Can you work these out from the model? Positions are in its coordinate system, mm. A direction names the side the tool comes from. Coordinates: 2 decimals unless noted, no trailing zeros. Write each loop counter-clockwise with the first axis right and the second up, starting at its lowest first coordinate (ties: lowest second). Pieces come first, ordered by that corner, then holes.
Solid Edge part; units mm, degrees
sketch "Sketch1" plane through (0, 0, 0) normal (1, 0, 0) x (0, 1, 0)
  line L0 (0, 0) -> (0, 35)
  line L1 (0, 35) -> (2, 35)
  line L2 (2, 35) -> (2, 0)
  line L3 (2, 0) -> (0, 0)
extrude "Protrusion1" add sketch "Sketch1" along normal mid plane 52
sketch "Sketch2" plane through (0, 0, 0) normal (1, 0, 0) x (0, 1, 0)
  line L0 (-55, 37) -> (0, 37)
  line L1 (2, 37) -> (0, 37)
  line L2 (2, 37) -> (2, 35)
  line L3 (0, 35) -> (2, 35)
  line L4 (0, 35) -> (-55, 35)
  line L5 (-55, 35) -> (-55, 37)
extrude "ExtrudedProtrusion_2" add sketch "Sketch2" along normal mid plane 125
sketch "Sketch3" plane through (0, -26.5, 37) normal (0, 0, 1) x (1, 0, 0)
  circle A0 centre (-52.3239, -17.6363) radius 2.5
  circle A1 centre (52.3239, -17.6363) radius 2.5
extrude "ExtrudedCutout_1" cut sketch "Sketch3" against normal blind 8.7921
sketch "Sketch4" plane through (0, 0, 17.5) normal (0, -1, 0) x (1, 0, 0)
  circle A0 centre (-19.7084, -11.8558) radius 2.5
  circle A1 centre (19.2978, -11.8558) radius 2.5
extrude "ExtrudedCutout_2" cut sketch "Sketch4" against normal blind 47.6347
sketch "Sketch5" plane through (0, 2, 18.5) normal (0, 1, 0) x (-1, 0, 0)
  line L0 (-28, -18.5) -> (-28, 16.5)
  line L1 (-28, 16.5) -> (-26, 16.5)
  line L2 (-26, 16.5) -> (-26, -18.5)
  line L3 (-26, -18.5) -> (-28, -18.5)
  line L4 (28, 16.5) -> (28, -18.5)
  line L5 (28, -18.5) -> (26, -18.5)
  line L6 (26, -18.5) -> (26, 16.5)
  line L7 (26, 16.5) -> (28, 16.5)
extrude "ExtrudedProtrusion_3" add sketch "Sketch5" against normal up to vertex (2 mm away) and the other way blind 15
fillet "Round_1" radius 5.06 2 edges at (28, 0, 17.5) (-28, 0, 17.5)
fillet "Round_2" radius 2 1 edges at (26, 2, 17.5)
fillet "Round_3" radius 2 1 edges at (-26, 2, 17.5)
fillet "Round_5" radius 2 2 edges at (25.4849, 2, 35) (-25.4849, 2, 35)
fillet "Round_6" radius 10 2 edges at (-62.5, -55, 36) (62.5, -55, 36)
1. I'm going to push flat-ended pins straight in: P1, Ø6, axis at y = -35, z = 30, coming from the +X side; P2, Ø4, axis at y = 9.5, z = 18, coming from the +X side; P3, Ø6, axis at x = 52.32, y = -44.14, coming from the -Z side; P4, Ø2, axis at x = -26.5, y = 12.5, coming from the +Z side. Where does each tip first touch, or does it pass through?
2. If we section it at B-B, the plane x = -19.5: List the corners of the cut face in (y, z) for me, plus the area to 3 significant figures.
3. We'd pull the mould along X, two halves only. Please class faces 1 (the face through (28, 11, 17)), 2 (the face through (-0.1, 1.6, 0)), 3 (the face through (-59.65, -51.99, 36.01)), 4 (the face through (-22.206, 0.986, 5.754)): released by +X, released by -X, zero draft, split by the parting line, or undercut.
4. Which directions (+Z, -Z, +X, -X, +Y, -Y) give clear straight access to the entire face, cutting with the end or side of a thin tool? Please do faces 5 (the face through (0, 0, 18)), 6 (the face through (-50.015, -45.094, 36.014)), 7 (the face through (-26, 11, 17)).
5. If I drill on L1, parallel to X at y = 9.5, z = 12; L2, parallel to X at y = 4, z = 29.5; L3, parallel to Z at x = -53.5, y = -25, over which ranges is the centre line in solid material (lowest first)?
6. If we section it at D-D, the plane x = 30: List the corners of the cut face in (y, z) for me, plus the area to 3 significant figures.
7. If we section it at C-C, the plane y = -5.5: List the corners of the cut face in (x, z) for me.
8. If we section it at A-A, the plane z = 25: List the corners of the cut face in (x, y) for me, plus the area to 3 significant figures.
Answers:
1. P1: passes through
1. P2: stops at x = 28
1. P3: stops at z = 35
1. P4: stops at z = 35
2. outline: (-55, 35) - (0, 35) - (0, 8.14) - (2, 8.14) - (2, 37) - (-55, 37) - close; (0, 0) - (2, 0) - (2, 3.15) - (0, 3.15) - close
2. area: 174 mm2
3. face 1: released by +X
3. face 2: zero draft
3. face 3: released by -X
3. face 4: undercut
4. face 5: -Z, +X, -X, -Y
4. face 6: +Z, -Z
4. face 7: +Z, -Z, +Y
5. L1: x = -28 to -26, 26 to 28
5. L2: x = -27.89 to -26, 26 to 27.89
5. L3: z = 35 to 37
6. outline: (-55, 35) - (2, 35) - (2, 37) - (-55, 37) - close
6. area: 114 mm2
7. outline: (-62.5, 35) - (62.5, 35) - (62.5, 37) - (-62.5, 37) - close
8. outline: (-28, 5.06) arc R5.06 ccw to (-22.94, 0) - (22.94, 0) arc R5.06 ccw to (28, 5.06) - (28, 17) - (26, 17) - (26, 4) arc R2 cw to (24, 2) - (-24, 2) arc R2 cw to (-26, 4) - (-26, 17) - (-28, 17) - close
8. area: 163 mm2
